Here's the drawing with two shaded views (mm, measured from the low corner). I have some questions. A direction names the side the tool comes from. Round coordinates to 2 decimals unless told otherwise and drop trailing zeros. Order: outer loops, then holes, each group sorted by start corner. A loop starts at its lowest first (then second) coordinate and runs counter-clockwise, first axis right, second up.
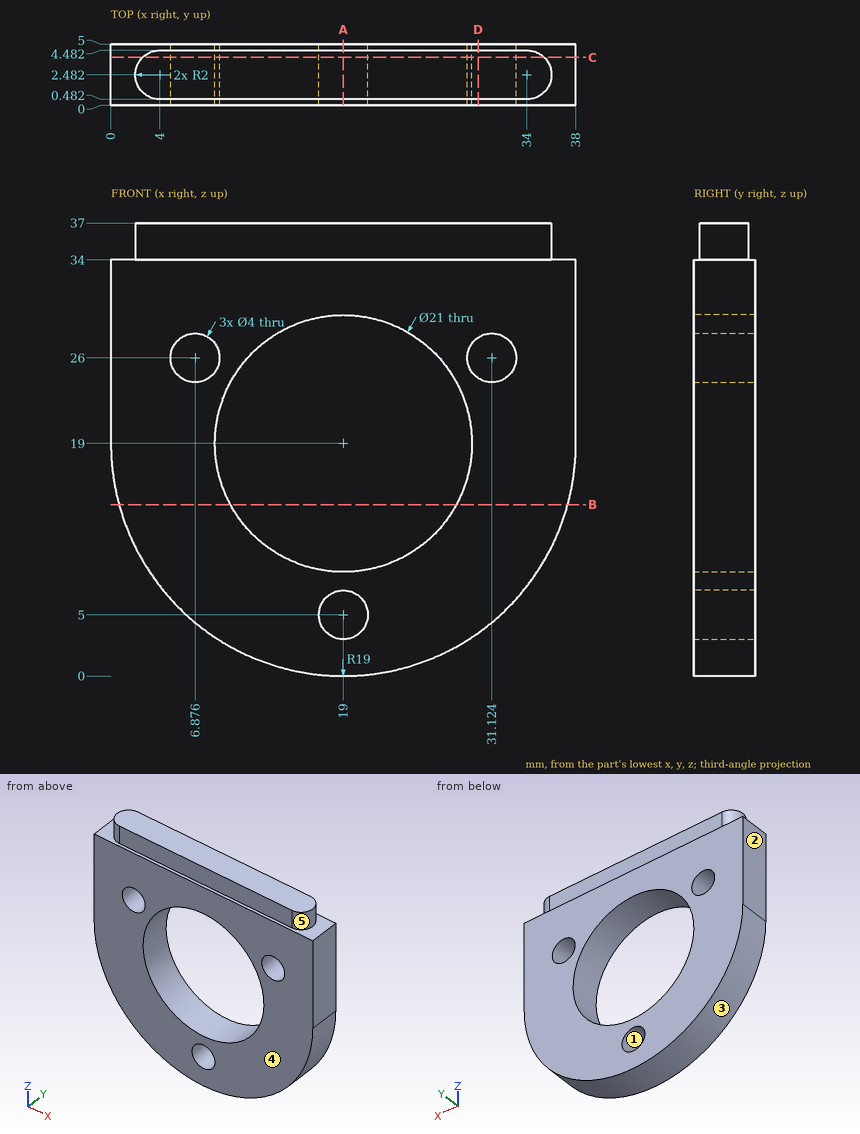
1. If we section it at D-D, the plane x = 30: Write out the boundary of the cut face in (y, z).
Evaluation:
outline: (0, 3.51) - (5, 3.51) - (5, 24.35) - (0, 24.35) - close; (0, 27.65) - (5, 27.65) - (5, 34) - (4.48, 34) - (4.48, 37) - (0.48, 37) - (0.48, 34) - (0, 34) - close
2. I need wall thicknesses on probe 1 along X at (y, z) = (1.15, 19); probe 2 along Z at (x, y) = (18, 3.3) (1 decimal); probe 3 along X at (y, z) = (3.9, 26) (1 decimal). Which ranges of each line are inside material? Lowest first, please.
Evaluation:
probe 1: x = 0 to 8.5, 29.5 to 38
probe 2: z = 0 to 3.3, 6.7 to 8.5, 29.5 to 37
probe 3: x = 0 to 4.9, 8.9 to 11.2, 26.8 to 29.1, 33.1 to 38
3. If we mould it in two halves opening along Z, with no side actions, what happens to the marked faces 1, 2 and 3? For each: released by +Z, released by -Z, zero draft, split by the parting line, or undercut.
Evaluation:
face 1: undercut
face 2: zero draft
face 3: released by -Z
4. If we section it at A-A, the plane x = 19: Write out the boundary of the cut face in (y, z).
Evaluation:
outline: (0, 0) - (5, 0) - (5, 3) - (0, 3) - close; (0, 7) - (5, 7) - (5, 8.5) - (0, 8.5) - close; (0, 29.5) - (5, 29.5) - (5, 34) - (4.48, 34) - (4.48, 37) - (0.48, 37) - (0.48, 34) - (0, 34) - close
5. If we section it at C-C, the plane y = 3.9: Write out the boundary of the cut face in (x, z) (1 decimal).
Evaluation:
outline: (0, 19) arc R19 ccw to (38, 19) - (38, 34) - (35.4, 34) - (35.4, 37) - (2.6, 37) - (2.6, 34) - (0, 34) - close; hole circle Ø4 at (6.9, 26); hole circle Ø21 at (19, 19); hole circle Ø4 at (19, 5); hole circle Ø4 at (31.1, 26)
6. On a 3-axis mill with a long thin cutter (end or side, diameter ignored), from which of +Z, -Z, +X, -X, +Y, -Y can I reach the whole of each face in a straight line? I mean the marked faces 4 and 5. Say none if no direction works.
Evaluation:
face 4: +Z, -Z, +X, -X, -Y
face 5: +Z, +X
7. If we section it at B-B, the plane z = 14: Write out the boundary of the cut face in (x, y).
Evaluation:
outline: (0.67, 0) - (9.77, 0) - (9.77, 5) - (0.67, 5) - close; (28.23, 0) - (37.33, 0) - (37.33, 5) - (28.23, 5) - close
8. I'm going to push flat-ended pins straight in: P1, Ø2, axis at y = 2, z = 17, coming from the -X side; P2, Ø3.5, axis at x = 24.5, z = 36, coming from the -Y side. Where does each tip first touch, or does it pass through?
Evaluation:
P1: stops at x = 0.03
P2: stops at y = 0.48
